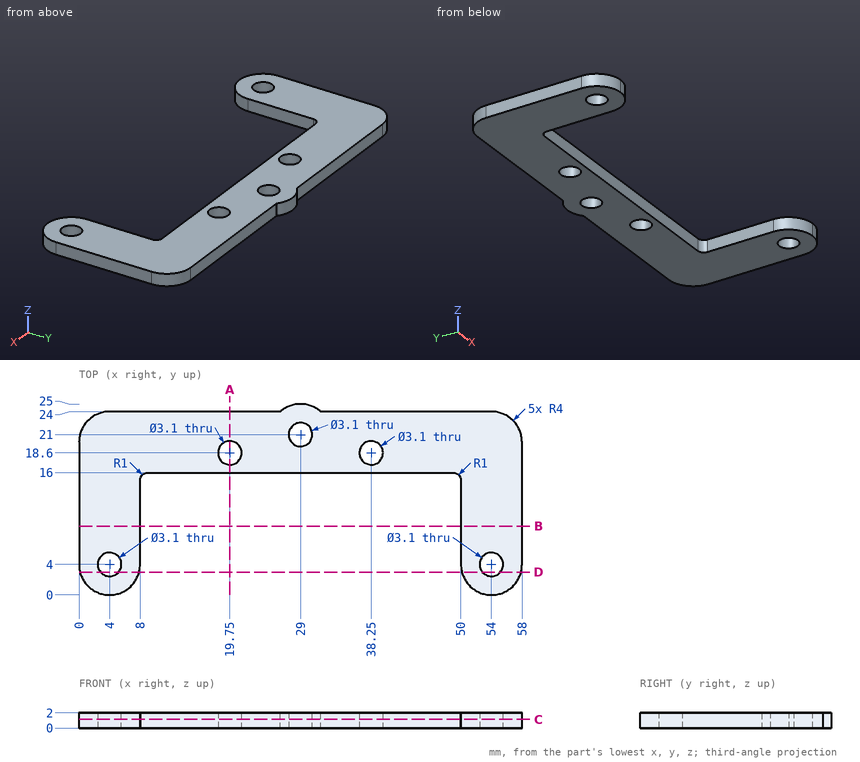
Job drawing, mm, ordinate dimensions from the low corner. One solid piece. Coordinates: 2 decimals unless noted, no trailing zeros. Order: outer loops, then holes, each group sorted by start corner. A loop starts at its lowest first (then second) coordinate and runs counter-clockwise, first axis right, second up. Notation, with made-up numbers: (-32, 17.5) - (-9, 17.5) arc R23 ccw to (-9, 53.5) - close; hole circle Ø2 at (42.25, 19). An arc over 180 degrees is marked (long way). Use CSV: the item, a comma, the result in double quotes.
Item 1: Saw through at A-A on x = 19.75. Give the cut face in (y, z), and give its area (3 significant figures).
Solved:
outline,"(16, 0) - (17.05, 0) - (17.05, 2) - (16, 2) - close; (20.15, 0) - (24, 0) - (24, 2) - (20.15, 2) - close"
area,"9.80 mm²"
Item 2: Saw through at C-C on z = 1.15. Give the cut face in (x, y).
Solved:
outline,"(0, 4) arc R4 ccw to (8, 4) - (8, 15) arc R1 cw to (9, 16) - (49, 16) arc R1 cw to (50, 15) - (50, 4) arc R4 ccw to (58, 4) - (58, 20) arc R4 ccw to (54, 24) - (31.65, 24) arc R4 ccw to (26.35, 24) - (4, 24) arc R4 ccw to (0, 20) - close; hole circle Ø3.1 at (4, 4); hole circle Ø3.1 at (19.75, 18.6); hole circle Ø3.1 at (29, 21); hole circle Ø3.1 at (38.25, 18.6); hole circle Ø3.1 at (54, 4)"
Item 3: Saw through at B-B on y = 9. Give the cut face in (x, z).
Solved:
outline,"(0, 0) - (8, 0) - (8, 2) - (0, 2) - close; (50, 0) - (58, 0) - (58, 2) - (50, 2) - close"
Item 4: Drop flat-ended pins along their axis: P1, Ø1, axis at x = 19.5, z = 1.5, coming from the -Y side; P2, Ø0.6, axis at x = 10, z = 1, coming from the +Y side. Give the stop position or say it passes through.
Solved:
P1,"stops at y = 16"
P2,"stops at y = 24"
Item 5: Probe probe 1 along X at (y, z) = (6.25, 1.65); probe 2 along X at (y, z) = (4.25, 0.15); probe 3 along Y at (x, z) = (29, 0.9). List the from-to ranges inside material, lowest first.
Solved:
probe 1,"x = 0 to 8, 50 to 58"
probe 2,"x = 0 to 2.47, 5.53 to 8, 50 to 52.47, 55.53 to 58"
probe 3,"y = 16 to 19.45, 22.55 to 25"
Item 6: Saw through at D-D on y = 3. Give the cut face in (x, z), and give its area (3 significant figures).
Solved:
outline,"(0.13, 0) - (2.82, 0) - (2.82, 2) - (0.13, 2) - close; (5.18, 0) - (7.87, 0) - (7.87, 2) - (5.18, 2) - close; (50.13, 0) - (52.82, 0) - (52.82, 2) - (50.13, 2) - close; (55.18, 0) - (57.87, 0) - (57.87, 2) - (55.18, 2) - close"
area,"21.5 mm²"
